Source: CAD feature listing. Evaluate the final solid. Frame: model axes, mm. A direction names the side the tool comes from. Coordinates: 2 decimals unless noted, no trailing zeros. Write each loop counter-clockwise with the first axis right and the second up, starting at its lowest first coordinate (ties: lowest second). Pieces come first, ordered by that corner, then holes. Notation, with made-up numbers: M 80,-7 L 89,-7 A20 cw 89,7 Z; hole C 31.25,46 d4. An arc over 180 degrees is marked long. Write item = value, one per line. Start each with the question number.
1. Line query: line 1 along X through (y, z) = (1, -1); line 2 along Z through (x, y) = (59.5, 1); line 3 along Z through (x, y) = (-6, 0.25). Output: solid intervals per line, ascending.
2. Access query for faces 1 (the face through (9, 3, 1)), 2 (the face through (7.5, 1, -38)), 3 (the face through (22.5, 1, -47)), 4 (the face through (22.5, 1, 47)), 5 (the face through (50.057, 1.521, -46.085)). Directions: +Z, -Z, +X, -X, +Y, -Y. A direction counts if a zero-diameter tool reaches every point of the face in a straight line with its end or side. Return the directions, or none.
3. Section query C-C (y = 1.5). Give the number of separate pieces and of enclosed holes in the cut face, then the cut area to 3 significant figures.
4. Section query A-A (z = -1.5). Output: boundary loops of the cut face in (x, y), then the cut area to 3 significant figures.
5. Pin query (flat end, axial travel): pin 1 Ø2 at (x, z) = (59.5, 29) entering from +Y; pin 2 Ø1.6 at (x, y) = (8.5, 1.5) entering from +Z; pin 3 Ø3 at (x, z) = (63.6, -7.21) entering from -Y; pin 4 Ø1.5 at (y, z) = (1, -47) entering from +X. Return the tip coordinate at first contact, or that it passes through.
6. Section query B-B (x = 59.5). Output: boundary loops of the cut face in (y, z), then the cut area to 3 significant figures.
7. Section query D-D (x = 2.5). Output: boundary loops of the cut face in (y, z), then the cut area to 3 significant figures.
8. Pull-direction query (X, two-part tool) for faces 6 (the face through (-32.357, 1.479, 0.707)), 7 (the face through (49.502, 1.521, 46.416)), 8 (the face through (16, 1, 1)); classes: pulls with the +X half, pulls with the -X half, needs draft (parallel to the pull), parting line crosses it, or undercut.
Autodesk Inventor part; units mm, degrees
ref_plane "YZ Plane" through (0, 0, 0) normal (1, 0, 0) x (0, 1, 0)
ref_plane "XZ Plane" through (0, 0, 0) normal (0, 1, 0) x (-1, 0, 0)
ref_plane "XY Plane" through (0, 0, 0) normal (0, 0, 1) x (1, 0, 0)
sketch "Boceto2" plane through (0, 0, 0) normal (0, 1, 0) x (-1, 0, 0)
  circle A0 centre (-10.65, 0) radius 62.5
  line L0 (-63, 32.5) -> (-63, -32.5)
  line L1 (-63, -32.5) -> (-33, -32.5)
  line L2 (-33, -32.5) -> (-33, 32.5)
  line L3 (-33, 32.5) -> (-63, 32.5)
  circle A1 centre (-59.5, -29) radius 1.25
  line L4 (0, 6.809) -> (0, -6.809)
  line L5 (10.65, 0) -> (-10.65, 0) construction
  circle A2 centre (-36.5, -29) radius 1.25
  circle A3 centre (-59.5, 29) radius 1.25
  circle A4 centre (-36.5, 29) radius 1.25
  line L6 (7.5, -42.3) -> (-7.5, -42.3)
  line L7 (-7.5, -42.3) -> (-7.5, -25)
  line L8 (-7.5, -25) -> (7.5, -25)
  line L9 (7.5, -25) -> (7.5, -42.3)
  arc A5 (9, -42.3) -> (9, -33.8) centre (9, -38.05) ccw
  line L10 (9, -42.3) -> (7.5, -42.3)
  line L11 (9, -33.8) -> (7.5, -33.8)
  arc A6 (9.5, -39.2) -> (9.5, -36.9) centre (9.5, -38.05) ccw
  line L12 (9.5, -39.2) -> (7.5, -39.2)
  line L13 (7.5, -39.2) -> (7.5, -36.9)
  line L14 (7.5, -36.9) -> (9.5, -36.9)
  line L15 (9.5, -36.9) -> (9.5, -39.2)
  arc A7 (-9, -33.8) -> (-9, -42.3) centre (-9, -38.05) ccw
  line L16 (-9, -42.3) -> (-7.5, -42.3)
  line L17 (-9, -33.8) -> (-7.5, -33.8)
  arc A8 (-9.5, -36.9) -> (-9.5, -39.2) centre (-9.5, -38.05) ccw
  line L18 (-9.5, -39.2) -> (-7.5, -39.2)
  line L19 (-7.5, -39.2) -> (-7.5, -36.9)
  line L20 (-7.5, -36.9) -> (-9.5, -36.9)
  line L21 (-9.5, -36.9) -> (-9.5, -39.2)
  line L22 (7.5, 42.3) -> (-7.5, 42.3)
  line L23 (-7.5, 42.3) -> (-7.5, 25)
  line L24 (-7.5, 25) -> (7.5, 25)
  line L25 (7.5, 25) -> (7.5, 42.3)
  arc A9 (9, 33.8) -> (9, 42.3) centre (9, 38.05) ccw
  line L26 (9, 42.3) -> (7.5, 42.3)
  line L27 (9, 33.8) -> (7.5, 33.8)
  arc A10 (9.5, 36.9) -> (9.5, 39.2) centre (9.5, 38.05) ccw
  line L28 (9.5, 39.2) -> (7.5, 39.2)
  line L29 (7.5, 39.2) -> (7.5, 36.9)
  line L30 (7.5, 36.9) -> (9.5, 36.9)
  line L31 (9.5, 36.9) -> (9.5, 39.2)
  line L32 (-9, 33.8) -> (-7.5, 33.8)
  line L33 (-7.5, 36.9) -> (-9.5, 36.9)
  line L34 (-7.5, 39.2) -> (-7.5, 36.9)
  line L35 (-9.5, 36.9) -> (-9.5, 39.2)
  line L36 (-9.5, 39.2) -> (-7.5, 39.2)
  arc A11 (-9.5, 39.2) -> (-9.5, 36.9) centre (-9.5, 38.05) ccw
  line L37 (-9, 42.3) -> (-7.5, 42.3)
  arc A12 (-9, 42.3) -> (-9, 33.8) centre (-9, 38.05) ccw
  line L38 (-16, -37.25) -> (-56, -37.25)
  line L39 (-56, -37.25) -> (-56, 37.25)
  line L40 (-56, 37.25) -> (-16, 37.25)
  line L41 (-16, 37.25) -> (-16, -37.25)
  line L42 (20.3604, -4.25) -> (0.1604, -4.25)
  line L43 (0.1604, -4.25) -> (0.1604, 4.25)
  line L44 (0.1604, 4.25) -> (20.3604, 4.25)
  line L45 (20.3604, 4.25) -> (20.3604, -4.25)
  line L46 (35.3604, -42.3) -> (-56.6604, -42.3)
  line L47 (-56.6604, -42.3) -> (-56.6604, 42.3)
  line L48 (-56.6604, 42.3) -> (35.3604, 42.3)
  line L49 (35.3604, 42.3) -> (35.3604, -42.3)
  line L50 (-67, -12.5) -> (-70, -12.5)
  line L51 (-70, -12.5) -> (-70, 12.5)
  line L52 (-70, 12.5) -> (-67, 12.5)
  line L53 (-67, 12.5) -> (-67, -12.5)
  line L54 (-19.3, -12.5) -> (-32, -12.5) construction
  line L55 (-32, -12.5) -> (-32, 7.82) construction
  line L56 (-32, 7.82) -> (-19.3, 7.82) construction
  line L57 (-19.3, 7.82) -> (-19.3, -12.5) construction
  line L58 (22.5, 52.3) -> (-22.5, 52.3)
  line L59 (-22.5, 52.3) -> (-22.5, 42.3)
  line L60 (-22.5, 42.3) -> (22.5, 42.3)
  line L61 (22.5, 42.3) -> (22.5, 52.3)
  line L62 (22.5, -52.3) -> (-22.5, -52.3)
  line L63 (-22.5, -52.3) -> (-22.5, -42.3)
  line L64 (-22.5, -42.3) -> (22.5, -42.3)
  line L65 (22.5, -42.3) -> (22.5, -52.3)
  line L66 (22.5, 52.3) -> (23.5693, 52.3)
  line L67 (-22.5, 52.3) -> (-44.8693, 52.3)
  line L68 (22.5, -52.3) -> (23.5693, -52.3)
  line L69 (-22.5, -52.3) -> (-44.8693, -52.3)
  circle A13 centre (-63.6, 6.2537) radius 1.15
  circle A14 centre (-63.6, -7.2083) radius 1.15
  arc A15 (23.5693, -52.3) -> (23.5693, 52.3) centre (-127.6415, 0) ccw
  point P0 (0, 0)
  point P1 (-33, 0)
  point P2 (0, 0)
  point P3 (13.25, -38.05)
  point P4 (10.65, -38.05)
  point P5 (-13.25, -38.05)
  point P6 (-10.65, -38.05)
  point P7 (13.25, 38.05)
  point P8 (10.65, 38.05)
  point P9 (-10.65, 38.05)
  point P10 (-13.25, 38.05)
  point P11 (-16, 0)
  point P12 (20.3604, 0)
  point P13 (-67, 0)
  point P14 (-56.6604, -42.3)
  point P15 (9, 42.3)
  point P16 (47.2734, 42.3)
  point P17 (0, 52.3)
  point P18 (-22.5, -42.3)
  point P19 (22.5, -42.3)
  point P20 (22.5, 42.3)
  dimension "d128" = 125
  dimension "d52" = 65
  dimension "d53" = 30
  dimension "d56" = 3.5
  dimension "d57" = 3.5
  dimension "d60" = 23
  dimension "d63" = 58
  dimension "d78" = 15
  dimension "d79" = 17.3
  dimension "d80" = 8.5
  dimension "d81" = 1.5
  dimension "d82" = 4.25
  dimension "d83" = 1.15
  dimension "d84" = 2.3
  dimension "d86" = 2
  dimension "d87" = 25
  dimension "d88" = 7.5
  dimension "d89" = 40
  dimension "d90" = 74.5
  dimension "d91" = 16
  dimension "d92" = 20.2
  dimension "d93" = 8.5
  dimension "d94" = 3
  dimension "d95" = 25
  dimension "d98" = 11
  dimension "d99" = 12.7
  dimension "d100" = 20.32
  dimension "d101" = 1
  dimension "d102" = 20
  dimension "d108" = 10
  dimension "d113" = 45
  dimension "d114" = 13.462
  dimension "d115" = 3.4
  dimension "d116" = 2.3
  dimension "d119" = 2.3
  dimension "d120" = 33
  dimension "d122" = 160
  dimension "d127" = 15
  dimension "d133" = 10.65
extrude "Extrusión4" add sketch "Boceto2" along normal blind 3 contours A0 L49 | L48 A15 A0 | L49 L46 A15 L48 | A0 A15 L46 | L66 L58 L67 A0 | A15 L48 L61 L66 | A15 L46 A5 L11 L9 L8 L7 L17 A7 L47 L1 L39 L38 L41 L40 L3 L48 A12 L32 L23 L24 L25 L27 A9 | A0 L69 L62 L68 | L68 L65 L46 A15 | L67 L59 L48 A0 | L61 L48 L26 L22 L37 L59 L58 | A0 L46 L63 L69 | L62 L63 L46 L16 L6 L10 L65 | L47 L3 L0 A13 A14 L1 A0 | A9 L27 L25 L30 A10 L28 L26 | L10 L9 L12 A6 L14 L11 A5 | L47 L1 L0 A14 A13 L3 | L3 L39 L1 L47 | L25 L24 L23 L22 | L6 L7 L8 L9 | L39 L40 L41 L38 L1 L2 L3 | L3 L2 L1 L39 | L37 L23 L36 A11 L33 L32 A12 | L28 L31 L30 L25 | A7 L17 L7 L20 A8 L18 L16 | L9 L14 L15 L12 | A13 L0 | L0 A13 | L23 L33 L35 L36 | A10 L31 | A14 L0 | L0 A14 | L18 L21 L20 L7 | L15 A6 | L35 A11 | A8 L21 | A1 | A2 | A3 | A4 | L42 L43 L44 L45 | L50 L51 L52 L53
extrude "Extrusión9" cut sketch "Boceto2" along normal blind 3 contours A0 L49 | L48 A15 A0 | L49 L46 A15 L48 | A0 A15 L46 | L66 L58 L67 A0 | A0 L69 L62 L68 | L61 L48 L26 L22 L37 L59 L58 | L62 L63 L46 L16 L6 L10 L65 | L39 L40 L41 L38 L1 L2 L3 | L3 L2 L1 L39 | L28 L31 L30 L25 | L9 L14 L15 L12 | A13 L0 | L0 A13 | L23 L33 L35 L36 | A10 L31 | A14 L0 | L0 A14 | L18 L21 L20 L7 | L15 A6 | L35 A11 | A8 L21 | A1 | A2 | A3 | A4 | L50 L51 L52 L53
fillet "Empalme6" radius 1 10 edges at (-23.5693, 1.5, 52.3) (-22.5, 1.5, 52.3) (-23.5693, 1.5, -52.3) (-22.5, 1.5, -52.3) (22.5, 1.5, -52.3) (22.5, 1.5, 52.3) (22.5, 1.5, -42.3) (-22.5, 1.5, -42.3) (-22.5, 1.5, 42.3) (22.5, 1.5, 42.3)
fillet "Empalme7" radius 43 2 edges at (44.8693, 1.5, 52.3) (44.8693, 1.5, -52.3)
properties part number "Parte inferior 2 v2" material "Madera (nogal)"
Results are:
q1.line_1 = -32.36 to 16, 56 to 67, 70 to 73.14
q1.line_2 = -38.34 to -30.25, -27.75 to 27.75, 30.25 to 38.34
q1.line_3 = -42.3 to 42.3
q2.face_1 = +Z, -Z, +X, -X, +Y
q2.face_2 = +Y, -Y
q2.face_3 = -Z, +Y, -Y
q2.face_4 = +Z, +Y, -Y
q2.face_5 = -Z, +X, +Y, -Y
q3.separate_pieces = 1
q3.enclosed_holes = 10
q3.area = 5,750 mm^2
q4.outline = M -32.35,0 L 16,0 L 16,3 L -32.35,3 Z; M 56,0 L 67,0 L 67,3 L 56,3 Z; M 70,0 L 73.13,0 L 73.13,3 L 70,3 Z
q4.area = 187 mm^2
q5.pin_1 = through
q5.pin_2 = 42.3
q5.pin_3 = 0
q5.pin_4 = 49.78
q6.outline = M 0,-38.34 L 3,-38.34 L 3,-30.25 L 0,-30.25 Z; M 0,-27.75 L 3,-27.75 L 3,27.75 L 0,27.75 Z; M 0,30.25 L 3,30.25 L 3,38.34 L 0,38.34 Z
q6.area = 215 mm^2
q7.outline = M 0,-42.3 L 3,-42.3 L 3,42.3 L 0,42.3 Z
q7.area = 254 mm^2
q8.face_6 = pulls with the -X half
q8.face_7 = pulls with the +X half
q8.face_8 = undercut
